Could you check a few things on this model? Use its own coordinates, in mm. A direction names the side the tool comes from. Give positions to 0.01 mm unless a question says otherwise; leave off trailing zeros. Loops run counter-clockwise (first coordinate to the right, second up) from the corner with the lowest first, then second, coordinate; pieces in that order, holes last. Notation, with made-up numbers: M -23.5,12.5 L -1.5,12.5 A14 ccw -1.5,24.5 Z; hole C 48.5,31 d10. An arc over 180 degrees is marked long. Answer in a Markdown table with one row per item. Add a question column.
1. If we section it at A-A on y = 6.5: List the corners of the cut face in (x, z) for me (3 decimals).
2. If we section it at D-D on z = -30: List the corners of the cut face in (x, y) for me (3 decimals), then the cut area to 3 significant figures.
3. I need wall thicknesses on line 1 along X through (y, z) = (13.25, -1.5) (3 decimals); line 2 along Z through (x, y) = (43, 1.75); line 3 along Z through (x, y) = (-12.5, 5.75). Which ranges of each line are inside material? Lowest first, please. Write a range as from..to.
4. If we section it at B-B on z = -12: List the corners of the cut face in (x, y) for me (3 decimals), then the cut area to 3 significant figures.
5. If we section it at C-C on x = 21: List the corners of the cut face in (y, z) for me.
6. Which directions (+Z, -Z, +X, -X, +Y, -Y) give clear straight access to the entire face, cutting with the end or side of a thin tool? Please do faces 1 (the flat face through (51, 1, -16.002)), 2 (the flat face through (51, 1, 9.398)), 3 (the flat face through (-9.525, 4, -40)), 4 (the flat face through (51, 2.54, -3)).
7. I'm going to push flat-ended pins straight in: pin 1 Ø14 at (x, z) = (50, 0) entering from +Y; pin 2 Ø12 at (y, z) = (9, -21) entering from +X (3 decimals); pin 3 Ø17 at (x, z) = (-2, -38) entering from +Y. Where does each tip first touch, or does it pass through?
```python
from build123d import *

# Parameters (mm, degrees)
SKETCH1_W           = 85.09
SKETCH1_H           = 55.88
BOSS_EXTRUDE1_DEPTH = 24.13
SKETCH2_W           = 17.78
SKETCH2_H           = 25.4
BOSS_EXTRUDE2_DEPTH = 2.54
SKETCH3_W           = 15.24
SKETCH3_H           = 7.62
BOSS_EXTRUDE3_DEPTH = 25.4


with BuildPart() as part:
    # Sketch1 → Boss-Extrude1 (new body)
    with BuildSketch(Plane(origin=(0, 0, 0), x_dir=(1, 0, 0), z_dir=(0, 1, 0))):
        Rectangle(SKETCH1_W, SKETCH1_H)
    extrude(amount=BOSS_EXTRUDE1_DEPTH)

    # Sketch2 → Boss-Extrude2 (add)
    with BuildSketch(Plane.XZ):
        with Locations((51.435, -3.302)):
            Rectangle(SKETCH2_W, SKETCH2_H)
    extrude(amount=-BOSS_EXTRUDE2_DEPTH)

    # Sketch3 → Boss-Extrude3 (add)
    with BuildSketch(Plane(origin=(0, 0, -27.94), x_dir=(-1, 0, 0), z_dir=(0, 0, -1))):
        with Locations((1.905, 3.81)):
            Rectangle(SKETCH3_W, SKETCH3_H)
    extrude(amount=BOSS_EXTRUDE3_DEPTH)


solid = part.part
```
Results:
| question | item | result |
|---|---|---|
| 1 | outline | M -42.545,-27.94 L -9.525,-27.94 L -9.525,-53.34 L 5.715,-53.34 L 5.715,-27.94 L 42.545,-27.94 L 42.545,27.94 L -42.545,27.94 Z |
| 2 | outline | M -9.525,0 L 5.715,0 L 5.715,7.62 L -9.525,7.62 Z |
| 2 | area | 116 mm2 |
| 3 | line 1 | -42.545..42.545 |
| 3 | line 2 | -16..9.4 |
| 3 | line 3 | -27.94..27.94 |
| 4 | outline | M -42.545,0 L 60.325,0 L 60.325,2.54 L 42.545,2.54 L 42.545,24.13 L -42.545,24.13 Z |
| 4 | area | 2,100 mm2 |
| 5 | outline | M 0,-27.94 L 24.13,-27.94 L 24.13,27.94 L 0,27.94 Z |
| 6 | face 1 | -Z, +X, +Y, -Y |
| 6 | face 2 | +Z, +X, +Y, -Y |
| 6 | face 3 | -Z, -X, +Y, -Y |
| 6 | face 4 | +Z, -Z, +X, +Y |
| 7 | pin 1 | y = 2.54 |
| 7 | pin 2 | x = 42.545 |
| 7 | pin 3 | y = 7.62 |
